from build123d import *

# Parameters (mm, degrees)
SKETCH1_W                   = 82
SKETCH1_H                   = 50
BOSS_EXTRUDE1_DEPTH         = 16
CHAMFER1_SIZE               = 1.5
CHAMFER2_SIZE               = 1.5
CHAMFER3_SIZE               = 1.5
CHAMFER4_SIZE               = 1.5
M4_TAPPED_HOLE4_D           = 3.3
M4_TAPPED_HOLE4_DEPTH       = 8
M4_TAPPED_HOLE4_CSINK_D     = 4.05
M4_TAPPED_HOLE4_CSINK_ANGLE = 100
M4_TAPPED_HOLE4_TIP         = 0.991420021


with BuildPart() as part:
    # Sketch1 → Boss-Extrude1 (new body)
    with BuildSketch(Plane(origin=(0, 0, 0), x_dir=(1, 0, 0), z_dir=(0, 1, 0))):
        Rectangle(SKETCH1_W, SKETCH1_H)
    extrude(amount=BOSS_EXTRUDE1_DEPTH)

    # Chamfer1
    chamfer1_edges = [part.edges().sort_by_distance(p)[0] for p in [
        (-41, 16, 0),
    ]]
    chamfer(chamfer1_edges, length=CHAMFER1_SIZE)

    # Chamfer2
    chamfer2_edges = [part.edges().sort_by_distance(p)[0] for p in [
        (0.75, 16, 25),
    ]]
    chamfer(chamfer2_edges, length=CHAMFER2_SIZE)

    # Chamfer3
    chamfer3_edges = [part.edges().sort_by_distance(p)[0] for p in [
        (41, 16, -0.75),
    ]]
    chamfer(chamfer3_edges, length=CHAMFER3_SIZE)

    # Chamfer4
    chamfer4_edges = [part.edges().sort_by_distance(p)[0] for p in [
        (0, 16, -25),
    ]]
    chamfer(chamfer4_edges, length=CHAMFER4_SIZE)

    # M4 Tapped Hole4
    with Locations(Plane(origin=(0, 16, 0), x_dir=(1, 0, 0), z_dir=(0, 1, 0))):
        with Locations((-19, 12.5), (19, 12.5), (19, -12.5), (-19, -12.5)):
            CounterSinkHole(M4_TAPPED_HOLE4_D / 2, M4_TAPPED_HOLE4_CSINK_D / 2, depth=M4_TAPPED_HOLE4_DEPTH, counter_sink_angle=M4_TAPPED_HOLE4_CSINK_ANGLE)
            with Locations((0, 0, -(M4_TAPPED_HOLE4_DEPTH + M4_TAPPED_HOLE4_TIP / 2))):  # 118° drill point
                Cone(0, M4_TAPPED_HOLE4_D / 2, M4_TAPPED_HOLE4_TIP, mode=Mode.SUBTRACT)


solid = part.part
Input: part model. Units: mm. Frame: model coordinates. A direction names the side the tool comes from. Round coordinates to 2 decimals unless told otherwise and drop trailing zeros.
1. Pin query (flat end, axial travel): P1, Ø2.5, axis at x = 19, z = 12.5, coming from the +Y side; P2, Ø3, axis at x = -19, z = 12.5, coming from the +Y side. Return the tip coordinate at first contact, or that it passes through.
The answers:
P1: stops at y = 7.76
P2: stops at y = 7.91
2. Mould query, pull axis Z, two halves, no side actions, for faces 3 (the face through (-0.6, 15.3, 24.2)), 4 (the face through (20.31, 11.79, 13.5)), 5 (the face through (-1, 7, -25)). Classes: released by +Z, released by -Z, zero draft, split by the parting line, or undercut.
The answers:
face 3: released by +Z
face 4: undercut
face 5: released by -Z
3. Set-up query: faces 1 (the face through (41, 7, 0)), 2 (the face through (-17.69, 11.79, -11.5)). Return all of +Z, -Z, +X, -X, +Y, -Y with unobstructed straight access to the full face (end or side cutting, diameter ignored); none if empty.
The answers:
face 1: +Z, -Z, +X, +Y, -Y
face 2: +Y
4. Material intervals for line 1 (Z direction, x = -19, y = 13); line 2 (X direction, y = 12.5, z = 12.5); line 3 (Y direction, x = 20, z = -11), sorted ascending.
The answers:
line 1: z = -25 to -14.15, -10.85 to 10.85, 14.15 to 25
line 2: x = -41 to -20.65, -17.35 to 17.35, 20.65 to 41
line 3: y = 0 to 15.81
